Geometry check sheet. Reference: the model listing, model coordinates, mm. Give positions to 0.01 mm unless a question says otherwise; leave off trailing zeros. Loops run counter-clockwise (first coordinate to the right, second up) from the corner with the lowest first, then second, coordinate; pieces in that order, holes last. Notation, with made-up numbers: (27, 60.25) -> (60, 60.25) arc R16 cw to (60, 91.25) -> close; hole circle Ø9 at (42, 83.5). An arc over 180 degrees is marked (long way). One line per question, with ' | ' between items.
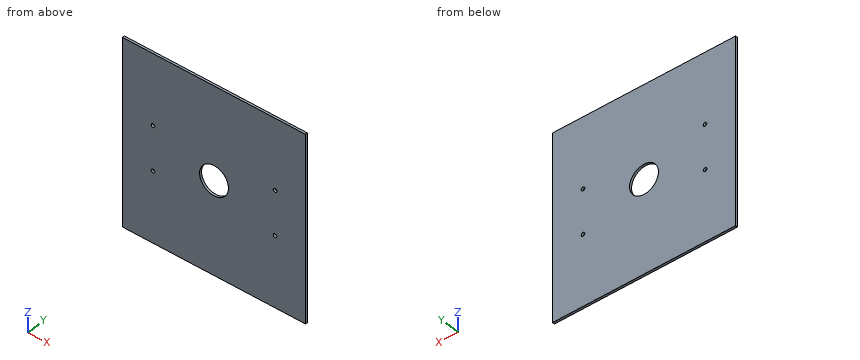
Autodesk Inventor part; units mm, degrees
ref_plane "YZ Plane" through (0, 0, 0) normal (1, 0, 0) x (0, 1, 0)
ref_plane "XZ Plane" through (0, 0, 0) normal (0, 1, 0) x (-1, 0, 0)
ref_plane "XY Plane" through (0, 0, 0) normal (0, 0, 1) x (1, 0, 0)
sketch "Sketch1" plane through (0, 0, 0) normal (0, 1, 0) x (-1, 0, 0)
  line L0 (126.9625, -125.6) -> (-126.9625, -125.6)
  line L1 (-126.9625, -125.6) -> (-126.9625, 125.6)
  line L2 (-126.9625, 125.6) -> (126.9625, 125.6)
  line L3 (126.9625, 125.6) -> (126.9625, -125.6)
  line L4 (126.9625, -125.6) -> (-126.9625, 125.6) construction
  line L5 (-126.9625, -125.6) -> (126.9625, 125.6) construction
  point P0 (0, 0)
  dimension "d0" = 253.925
  dimension "d1" = 251.2
extrude "Extrusion1" add sketch "Sketch1" along normal blind 3.15
sketch "Sketch4" plane through (0, 0, 0) normal (0, -1, 0) x (1, 0, 0)
  line L0 (-126.9625, 125.6) -> (-126.9625, -125.6)
  line L1 (126.9625, -40) -> (-126.9625, -40)
  line L2 (-126.9625, -40) -> (-126.9625, 40)
  line L3 (-126.9625, 40) -> (126.9625, 40)
  line L4 (126.9625, 40) -> (126.9625, -40)
  line L5 (126.9625, -40) -> (-126.9625, 40) construction
  line L6 (-126.9625, -40) -> (126.9625, 40) construction
  circle A0 centre (-84.6417, 30) radius 2.5
  line L7 (0, 0) -> (-126.9625, 0)
  line L8 (-126.9625, 0) -> (-126.9625, 40)
  line L9 (-126.9625, 40) -> (0, 40)
  line L10 (0, 40) -> (0, 0)
  circle A1 centre (-84.6417, -30) radius 2.5
  circle A2 centre (84.6417, 30) radius 2.5
  circle A3 centre (84.6417, -30) radius 2.5
  circle A4 centre (0, 0) radius 20
  dimension "d20" = 80
  dimension "d21" = 5
  dimension "d22" = 10
  dimension "d23" = 84.6417
  dimension "d24" = 40
extrude "Extrusion4" cut sketch "Sketch4" against normal up to next contours A4 L10 L7 | L7 L10 A4 | A0 | A1 | A2 | A3
equation "\"d0\" = visor_x"
equation "\"d1\" = 2 * visor_y + frame_y"
equation "\"d2\" = clear_acrylic"
equation "\"d20\" = frame_y"
equation "\"d21\" = m5_diameter"
equation "\"d22\" = 0.5 * visor_overlap"
equation "\"d23\" = 0.333333 * visor_x"
equation "\"d24\" = 0.5 * frame_y"
equation "\"sm_thickness\" = 1.5875"
equation "\"very_thick_acrylic\" = 9.45"
equation "\"thick_acrylic\" = 5.88"
equation "\"thin_acrylic\" = 3.15"
equation "\"clear_acrylic\" = 3.15"
equation "\"wood_thickness\" = 6.72"
equation "\"m3_diameter\" = 3"
equation "\"m4_diameter\" = 4"
equation "\"m5_diameter\" = 5"
equation "\"brass_insert_drill\" = 4"
equation "\"m5_brass_insert_drill\" = 6.7"
equation "\"m3_main_length\" = 14"
equation "\"m3_main_nut_width\" = 5.7"
equation "\"m3_main_nut_thickness\" = 2.5"
equation "\"m3_main_extra\" = 1"
equation "\"stepper_screw_space\" = 35"
equation "\"stepper_shaft_diameter\" = 5"
equation "\"stepper_body_diameter\" = 28"
equation "\"laser_body_diameter\" = 12"
equation "\"t_carrier\" = 5.88"
equation "\"t_wall\" = 5.88"
equation "\"t_window\" = 3.15"
equation "\"carrier_y\" = 251"
equation "\"carrier_z\" = 12"
equation "\"carrier_z2\" = 25"
equation "\"protection_slot\" = 44.2"
equation "\"protection_slot_offset\" = 55.25"
equation "\"window_z\" = 332.225"
equation "\"window_y\" = 93.75"
equation "\"door_sensor\" = 35"
equation "\"reservoir_x\" = 201"
equation "\"reservoir_y\" = 201"
equation "\"linear_bearing_spacing\" = 271"
equation "\"motor_spacing\" = 337"
equation "\"t_tray\" = 3.15"
equation "\"tray_border\" = 25"
equation "\"tray_x\" = 251"
equation "\"tray_y\" = 251"
equation "\"bed_z\" = 25"
equation "\"brass_keep_out\" = 8"
equation "\"tape_keep_out\" = 2"
equation "\"tape_thickness\" = 2"
equation "\"t_crane\" = 6.72"
equation "\"crane_z2\" = 12"
equation "\"end_stop_spacing\" = 19"
equation "\"thumb_nut_offset_y\" = 0"
equation "\"thumb_nut_diameter\" = 7"
equation "\"z_min_from_center\" = 115"
equation "\"t_frame\" = 6.72"
equation "\"frame_top_z\" = 385"
equation "\"frame_bottom_z\" = 275"
equation "\"frame_total_z\" = 661.5875"
equation "\"frame_y\" = 80"
equation "\"frame_border\" = 48.0375"
equation "\"frame_foot_z\" = 12"
equation "\"frame_tilt\" = 1deg"
equation "\"printer_z\" = 289"
equation "\"lcd_x\" = 72"
equation "\"lcd_y\" = 25"
equation "\"subframe_x\" = 66"
equation "\"subframe_y_offset\" = 27.5"
equation "\"laser_y_offset\" = 19.4"
equation "\"laser_diameter\" = 12"
equation "\"laser_z_offset\" = 55"
equation "\"laser_y\" = 15"
equation "\"laser_z\" = 75"
equation "\"t_galvo_frame\" = 6.72"
equation "\"galvo_frame_x\" = 66"
equation "\"galvo_frame_z\" = 85"
equation "\"galvo_frame_y_offset\" = 27.5"
equation "\"drawer_x\" = 257.3"
equation "\"drawer_y\" = 90.3375"
equation "\"drawer_z\" = 278.175"
equation "\"drawer_z_from_bottom\" = 25"
equation "\"nema17_x\" = 43"
equation "\"visor_y\" = 85.6"
equation "\"visor_x\" = 253.925"
equation "\"door_z\" = 332.225"
equation "\"door_x\" = 251"
equation "\"window_overlap\" = 48"
equation "\"door_overlap\" = 48"
equation "\"acrylic_into_frame\" = 5"
equation "\"m3_press_nut_drill\" = 4.5"
equation "\"m3_head\" = 6"
equation "\"m5_head\" = 10.3"
equation "\"m5_press_nut_drill\" = 6.5"
equation "\"drawer_support_from_top\" = 48"
equation "\"laser_gap\" = 1"
equation "\"frame_screw_from_center\" = 25"
equation "\"drawer_screw_from_center\" = 55"
equation "\"frame_face_y\" = 45"
equation "\"switch_spacing\" = 19"
equation "\"subframe_y\" = 55"
equation "\"al_thickness\" = 1.5875"
equation "\"rivet_diameter\" = 3.3"
equation "\"bend_factor\" = 2.26205"
equation "\"al_bend\" = 3.591"
equation "\"sm_bend\" = 3.591"
equation "\"frame_x\" = 353.375"
equation "\"carrier_y2\" = 76.825"
properties part number "visor"
Item 1: Sectioned sample at C-C (y = 1.45). Record the cut outline in (x, z).
Result:
outline: (-126.96, -125.6) -> (126.96, -125.6) -> (126.96, 125.6) -> (-126.96, 125.6) -> close; hole circle Ø5 at (-84.64, -30); hole circle Ø5 at (-84.64, 30); hole circle Ø40 at (0, 0); hole circle Ø5 at (84.64, -30); hole circle Ø5 at (84.64, 30)
Item 2: Sectioned sample at B-B (x = 0). Record the cut outline in (y, z).
Result:
outline: (0, -125.6) -> (3.15, -125.6) -> (3.15, -20) -> (0, -20) -> close; (0, 20) -> (3.15, 20) -> (3.15, 125.6) -> (0, 125.6) -> close
Item 3: Scan line: probe 1 along Z at (x, y) = (9.5, 0.35). Record every from-to range of solid material in increasing order.
Result:
probe 1: -125.6 to -17.6, 17.6 to 125.6
Item 4: Sectioned sample at A-A (z = 0). Record the cut outline in (x, y), plus the area to 3 significant figures.
Result:
outline: (-126.96, 0) -> (-20, 0) -> (-20, 3.15) -> (-126.96, 3.15) -> close; (20, 0) -> (126.96, 0) -> (126.96, 3.15) -> (20, 3.15) -> close | area: 674 mm2
Item 5: Depth check by flat-ended pin: pin 1 Ø4.5 at (x, z) = (84.64, 30) entering from -Y; pin 2 Ø10 at (x, z) = (-57.5, -18) entering from -Y. Enter the tip coordinate at first touch or a pass-through.
Result:
pin 1: through | pin 2: y = 0
